from build123d import *

# Parameters (mm, degrees)
ESQUISSE1_R             = 2
BOSS_EXTRU_1_DEPTH      = 2
BOSS_EXTRU_2_DEPTH      = 45
ENL_V_MAT_EXTRU_2_REACH = 70.68
ESQUISSE4_R             = 10.5
BOSS_EXTRU_3_DEPTH      = 1
ENL_V_MAT_EXTRU_3_REACH = 74.062
ESQUISSE5_R             = 7
CONG_1_R                = 10


with BuildPart() as part:
    # Esquisse1 → Boss.-Extru.1 (new body)
    with BuildSketch(Plane.XY):
        Polygon((30, 40.1), (21, 40.1), (21, 9.9), (30, 9.9), (30, 0), (0, 0), (0, 50), (30, 50), align=None)
        with Locations((15, 45)):
            Circle(ESQUISSE1_R, mode=Mode.SUBTRACT)
        with Locations((15, 5)):
            Circle(ESQUISSE1_R, mode=Mode.SUBTRACT)
    extrude(amount=BOSS_EXTRU_1_DEPTH)

    # Esquisse2 → Boss.-Extru.2 (add)
    with BuildSketch(Plane.XY.offset(2)):
        Polygon((18, 40.1), (0, 40.1), (0, 37.1), (18, 37.1), (18, 12.9), (0, 12.9), (0, 9.9), (18, 9.9), (21, 9.9), (21, 40.1), align=None)
    extrude(amount=BOSS_EXTRU_2_DEPTH)

    # Enlèv. mat.-Extru.2: up to this face of the body (flat: up to its plane)
    enl_v_mat_extru_2_end = Plane(part.part.faces().sort_by_distance((10.5, 40.1, 24.5))[0])
    # Esquisse3 → Enlèv. mat.-Extru.2 (cut, up to the picked face)
    with BuildSketch(Plane.XZ.offset(-9.9), mode=Mode.PRIVATE) as enl_v_mat_extru_2_sk1:
        Polygon((0, 2), (18, 47), (0, 47), align=None)
    enl_v_mat_extru_2_tool1 = split(extrude(enl_v_mat_extru_2_sk1.sketch, amount=-ENL_V_MAT_EXTRU_2_REACH, mode=Mode.PRIVATE), bisect_by=enl_v_mat_extru_2_end, keep=Keep.BOTH, mode=Mode.PRIVATE)
    add(enl_v_mat_extru_2_tool1.solids().sort_by(Axis((6, 9.9, 32), (0, 1, 0)))[0], mode=Mode.SUBTRACT)

    # Esquisse4 → Boss.-Extru.3 (add)
    with BuildSketch(Plane(origin=(21, 0, 0), x_dir=(0, 0, -1), z_dir=(1, 0, 0))):
        with Locations(Location((-25, 25, 0), (0, 0, 270))):
            Circle(ESQUISSE4_R)
    extrude(amount=BOSS_EXTRU_3_DEPTH)

    # Esquisse5 → Enlèv. mat.-Extru.3 (cut, up to next)
    with BuildSketch(Plane(origin=(22, 0, 0), x_dir=(0, 0, -1), z_dir=(1, 0, 0)), mode=Mode.PRIVATE) as enl_v_mat_extru_3_sk1:
        with Locations(Location((-25, 25, 0), (0, 0, 90))):
            Circle(ESQUISSE5_R)
    enl_v_mat_extru_3_tool1 = extrude(enl_v_mat_extru_3_sk1.sketch, amount=-ENL_V_MAT_EXTRU_3_REACH, mode=Mode.PRIVATE) & part.part
    add(enl_v_mat_extru_3_tool1.solids().sort_by_distance((22, 25, 25))[0], mode=Mode.SUBTRACT)

    # Congé1
    # the kernel refuses this fillet: 10 mm, written as the material it takes off along each edge
    with BuildSketch(Plane(origin=(-7, 40.1, 47), x_dir=(0, 0, -1), z_dir=(1, 0, 0))) as cong_1_piece_1:
        with BuildLine():
            CenterArc((CONG_1_R, -CONG_1_R), CONG_1_R, 90, 90)
            Line((0, -CONG_1_R), (0, 0))
            Line((0, 0), (CONG_1_R, 0))
        make_face()
    extrude(amount=53, mode=Mode.SUBTRACT)
    with BuildSketch(Plane(origin=(46, 9.9, 47), x_dir=(0, 1, 0), z_dir=(-1, 0, 0))) as cong_1_piece_2:
        with BuildLine():
            CenterArc((CONG_1_R, CONG_1_R), CONG_1_R, 180, 90)
            Line((0, CONG_1_R), (0, 0))
            Line((0, 0), (CONG_1_R, 0))
        make_face()
    extrude(amount=53, mode=Mode.SUBTRACT)


solid = part.part
The listing builds one solid part. Answer for the finished solid, in the listing's coordinates (mm). A direction names the side the tool comes from. Coordinates: 2 decimals unless noted, no trailing zeros. Order: outer loops, then holes, each group sorted by start corner. A loop starts at its lowest first (then second) coordinate and runs counter-clockwise, first axis right, second up. Notation, with made-up numbers: (-33.5, -38.5) -> (-13.5, -38.5) arc R5 ccw to (-13.5, -30.5) -> close; hole circle Ø8 at (-9, -17.5). An arc over 180 degrees is marked (long way). Answer in a Markdown table with one row per item. Add a question column.
Item 1: Find section B-B (z = 25). Write down the section's boundary in (x, y), then the cut area to 3 significant figures.
Item 2: Find the intervals of material crossed by L1, parallel to Y at x = 15, z = 1.55; L2, parallel to Z at x = 3, y = 7.5; L3, parallel to X at y = 21.5, z = 6, in increasing order. Write a range as from..to.
Item 3: Determine the mould class of faces 4 (the face through (20.028, 23.483, 18.166)), 5 (the face through (18.23, 38.35, 42.65)), 6 (the face through (15, 50, 1)) for opening direction Z: +Z half, -Z half, draft (parallel to the pull), parting line (faces both ways), or undercut.
Item 4: Which of the six approach directions +Z, -Z, +X, -X, +Y, -Y give full straight-line access (tool end or side, diameter ignored) to faces 1 (the face through (15.2, 47.3, 2)), 2 (the face through (21.493, 32.739, 17.904)), 3 (the face through (9, 25, 2))?
Item 5: Each of these flat-tipped pins is pushed along its axis until it touches: P1, Ø9, axis at x = 7.5, y = 26, coming from the +Z side; P2, Ø1.5, axis at y = 40, z = 8.5, coming from the +X side; P3, Ø6.5, axis at x = 7.5, z = 11, coming from the +Y side; P4, Ø1, axis at x = 4.5, y = 17, coming from the -Z side. Where does it stop, or does it pass through?
Item 6: Find section C-C (x = 19). Write down the section's boundary in (y, z).
Item 7: Find section A-A (y = 45). Write down the section's boundary in (x, z), then the cut area to 3 significant figures.
Item 8: Find section D-D (x = 26.5). Write down the section's boundary in (y, z), then the cut area to 3 significant figures.
Result set:
| question | item | result |
|---|---|---|
| 1 | outline | (9.2, 9.9) -> (21, 9.9) -> (21, 14.5) -> (22, 14.5) -> (22, 18) -> (18, 18) -> (18, 12.9) -> (9.2, 12.9) -> close; (9.2, 37.1) -> (18, 37.1) -> (18, 32) -> (22, 32) -> (22, 35.5) -> (21, 35.5) -> (21, 40.1) -> (9.2, 40.1) -> close |
| 1 | area | 108 mm² |
| 2 | L1 | y = 0..3, 7..43, 47..50 |
| 2 | L2 | z = 0..2 |
| 2 | L3 | x = 18..21 |
| 3 | face 4 | undercut |
| 3 | face 5 | +Z half |
| 3 | face 6 | draft |
| 4 | face 1 | +Z, +X, -X, +Y |
| 4 | face 2 | +X |
| 4 | face 3 | +Z, -X |
| 5 | P1 | stops at z = 2 |
| 5 | P2 | stops at x = 21 |
| 5 | P3 | stops at y = 40.1 |
| 5 | P4 | stops at z = 0 |
| 6 | outline | (0, 0) -> (50, 0) -> (50, 2) -> (40.1, 2) -> (40.1, 37) arc R10 ccw to (30.1, 47) -> (19.9, 47) arc R10 ccw to (9.9, 37) -> (9.9, 2) -> (0, 2) -> close; hole circle Ø14 at (25, 25) |
| 7 | outline | (0, 0) -> (13, 0) -> (13, 2) -> (0, 2) -> close; (17, 0) -> (30, 0) -> (30, 2) -> (17, 2) -> close |
| 7 | area | 52.0 mm² |
| 8 | outline | (0, 0) -> (9.9, 0) -> (9.9, 2) -> (0, 2) -> close; (40.1, 0) -> (50, 0) -> (50, 2) -> (40.1, 2) -> close |
| 8 | area | 39.6 mm² |
